Autodesk Inventor part; units mm, degrees
ref_plane "YZ Plane" through (0, 0, 0) normal (1, 0, 0) x (0, 1, 0)
ref_plane "XZ Plane" through (0, 0, 0) normal (0, 1, 0) x (-1, 0, 0)
ref_plane "XY Plane" through (0, 0, 0) normal (0, 0, 1) x (1, 0, 0)
sketch "Esboço1" plane through (0, 0, 0) normal (0, 0, 1) x (1, 0, 0)
  line L0 (-7.5, 7.5) -> (7.5, 7.5) construction
  line L1 (-7.5, 7.5) -> (-7.5, 3.1) construction
  line L2 (-7.5, 3.1) -> (-5.5, 3.1) construction
  line L3 (-5.5, 6.1) -> (-5.5, 3.1) construction
  line L4 (-5.5, 6.1) -> (-1.5, 2.7436) construction
  line L5 (-1.5, 2.7436) -> (-1.5, 0) construction
  line L6 (-1.5, 0) -> (0, 0)
  line L7 (0, 0) -> (0, 7.5)
  arc A0 (-6.5, 7.5) -> (-7.5, 6.5) centre (-6.5, 6.5) ccw
  arc A1 (-4.6786, 5.4108) -> (-5.5, 5.0277) centre (-5, 5.0277) ccw
  arc A2 (-1.5, 2.2773) -> (-1.8572, 3.0433) centre (-2.5, 2.2773) ccw
  line L8 (-7.5, 3.1) -> (-7, 3.1) construction
  line L9 (-7, 3.1) -> (-7, 3.6)
  line L10 (-7, 3.6) -> (-7.5, 3.6)
  line L11 (-7.5, 3.6) -> (-7.5, 3.1) construction
  line L12 (-7.5, 6.5) -> (-7.5, 3.6)
  line L13 (-7, 3.1) -> (-5.5, 3.1)
  line L14 (-5.5, 5.0277) -> (-5.5, 3.1)
  line L15 (-4.6786, 5.4108) -> (-1.8572, 3.0433)
  line L16 (-1.5, 0) -> (-1.5, 2.2773)
  line L17 (-6.5, 7.5) -> (0, 7.5)
  point P0 (-7.5, 5.3)
  dimension "d0" = 15
  dimension "d2" = 7.5
  dimension "d3" = 3.1
  dimension "d4" = 2
  dimension "d5" = 3
  dimension "d6" = 6
  dimension "d7" = 50
  dimension "d10" = 1
  dimension "d11" = 0.5
  dimension "d12" = 1
  dimension "d13" = 0.5
extrude "Extrusão1" add sketch "Esboço1" along normal mid plane 100
mirror "Espelhar1" about plane through (0, 0, 0) normal (1, 0, 0) of "Extrusão1"
mirror "Espelhar2" about plane through (0, 0, 0) normal (0, 1, 0) of "Extrusão1", "Espelhar1"
properties part number "perfil_15x15_001" material "Alumínio 6061"
Build history of the part. All positions in model axes, mm. A direction names the side the tool comes from. Round coordinates to 2 decimals unless told otherwise and drop trailing zeros. Write each loop counter-clockwise with the first axis right and the second up, starting at its lowest first coordinate (ties: lowest second). Pieces come first, ordered by that corner, then holes. Notation, with made-up numbers: M -22.75,21.25 L 24.25,21.25 A11 ccw 24.25,37.25 Z; hole C -8.5,75.5 d9. An arc over 180 degrees is marked long. Answer in a Markdown table with one row per item.
1. Saw through at A-A (x = 3). List the corners of the cut face in (y, z).
Geometry check:
| item | result |
|---|---|
| outline | M -7.5,-50 L -4,-50 L -4,50 L -7.5,50 Z; M 4,-50 L 7.5,-50 L 7.5,50 L 4,50 Z |
2. Which spindle directions (+Z, -Z, +X, -X, +Y, -Y) get a long thin tool onto all of the face, cutting with end or side? Do faces 4 (the face through (-3, 4, -1)), 5 (the face through (-1.5, 0, -1)), 6 (the face through (1.5, 0, -1)). Say none if no direction does.
Geometry check:
| item | result |
|---|---|
| face 4 | +Z, -Z |
| face 5 | +Z, -Z, -X |
| face 6 | +Z, -Z, +X |
3. Mould opens along X. For faces 1 (the face through (0, 0, 50)), 2 (the face through (3, 4, -1)), 3 (the face through (7.5, 5, -1)) say: +X half, -X half, draft (parallel to the pull), parting line (faces both ways), or undercut.
Geometry check:
| item | result |
|---|---|
| face 1 | draft |
| face 2 | undercut |
| face 3 | +X half |
4. Probe L1, parallel to X at y = 4.5, z = 9; L2, parallel to X at y = -4, z = 13.5; L3, parallel to Y at x = -4, z = -25. List the from-to ranges inside material, lowest first. Write a range as [from, to].
Geometry check:
| item | result |
|---|---|
| L1 | [-7.5, -5.5], [-3.59, 3.59], [5.5, 7.5] |
| L2 | [-7.5, -5.5], [-3, 3], [5.5, 7.5] |
| L3 | [-7.5, -4.84], [4.84, 7.5] |
5. Flat gauge pins, fed straight in: P1, Ø0.6, axis at x = -7.5, z = -2, coming from the +Y side; P2, Ø3, axis at y = -1, z = 17.5, coming from the -X side; P3, Ø1.4, axis at y = 0, z = 10.5, coming from the +X side. Where does each tip first touch, or does it go through?
Geometry check:
| item | result |
|---|---|
| P1 | y = 7.21 |
| P2 | x = -1.53 |
| P3 | x = 1.5 |
6. Saw through at B-B (y = -0.75). List the corners of the cut face in (x, z), and give its area (3 significant figures).
Geometry check:
| item | result |
|---|---|
| outline | M -1.5,-50 L 1.5,-50 L 1.5,50 L -1.5,50 Z |
| area | 300 mm2 |
